Geometry: final body of the model. Coordinates: model frame, mm. Face numbers are marked on the shaded views. A direction names the side the tool comes from. Round coordinates to 2 decimals unless told otherwise and drop trailing zeros. Loops run counter-clockwise (first coordinate to the right, second up) from the corner with the lowest first, then second, coordinate; pieces in that order, holes last. Notation, with made-up numbers: M 27,-6 L 59,-6 A23 cw 59,29 Z; hole C 8,4.25 d9. An arc over 180 degrees is marked long. Write each question's results on one line, items separated by ' | '.
```python
from build123d import *

# Parameters (mm, degrees)
BOSS_EXTRUDE1_DEPTH = 40
SKETCH2_R           = 1.516102493
CUT_EXTRUDE1_DEPTH  = 10
SKETCH3_R           = 1.505855903
BOSS_EXTRUDE2_DEPTH = 5


with BuildPart() as part:
    # Sketch1 → Boss-Extrude1 (new body)
    with BuildSketch(Plane(origin=(0, 0, 0), x_dir=(1, 0, 0), z_dir=(0, 1, 0))):
        Polygon((0, -2.886751346), (2.5, -1.443375673), (2.5, 1.443375673), (0, 2.886751346), (-2.5, 1.443375673), (-2.5, -1.443375673), align=None)
    extrude(amount=BOSS_EXTRUDE1_DEPTH)

    # Sketch2 → Cut-Extrude1 (cut)
    with BuildSketch(Plane(origin=(0, 40, 0), x_dir=(1, 0, 0), z_dir=(0, 1, 0))):
        Circle(SKETCH2_R)
    extrude(amount=-CUT_EXTRUDE1_DEPTH, mode=Mode.SUBTRACT)

    # Sketch3 → Boss-Extrude2 (add)
    with BuildSketch(Plane.XZ):
        Circle(SKETCH3_R)
    extrude(amount=BOSS_EXTRUDE2_DEPTH)


solid = part.part
```
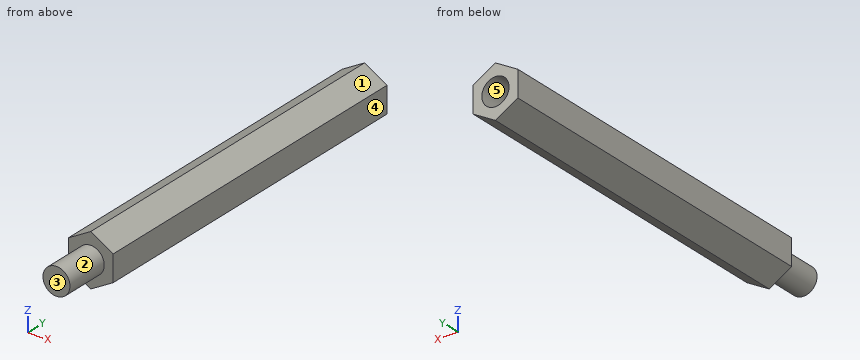
1. Draft query along X for the marked faces 3, 4 and 5. Return one class per face: pulls with the +X half, pulls with the -X half, needs draft (parallel to the pull), parting line crosses it, or undercut.
Answer key:
face 3: needs draft | face 4: pulls with the +X half | face 5: undercut
2. Section B-B (y = 31.5). Output: boundary loops of the cut face in (x, z).
Answer key:
outline: M -2.5,-1.44 L 0,-2.89 L 2.5,-1.44 L 2.5,1.44 L 0,2.89 L -2.5,1.44 Z; hole C 0,0 d3.03
3. Section A-A (z = 0). Output: boundary loops of the cut face in (x, y).
Answer key:
outline: M -2.5,0 L -1.51,0 L -1.51,-5 L 1.51,-5 L 1.51,0 L 2.5,0 L 2.5,40 L 1.52,40 L 1.52,30 L -1.52,30 L -1.52,40 L -2.5,40 Z
4. Section C-C (y = 21). Output: boundary loops of the cut face in (x, z).
Answer key:
outline: M -2.5,-1.44 L 0,-2.89 L 2.5,-1.44 L 2.5,1.44 L 0,2.89 L -2.5,1.44 Z
5. Pin query (flat end, axial travel): P1, Ø0.9, axis at x = -0.5, z = -0.5, coming from the +Y side; P2, Ø1, axis at x = -1, z = -2, coming from the -Y side. Return the tip coordinate at first contact, or that it passes through.
Answer key:
P1: stops at y = 30 | P2: stops at y = 0
6. Section D-D (x = -0.85). Output: boundary loops of the cut face in (y, z).
Answer key:
outline: M -5,-1.24 L 0,-1.24 L 0,-2.4 L 40,-2.4 L 40,-1.26 L 30,-1.26 L 30,1.26 L 40,1.26 L 40,2.4 L 0,2.4 L 0,1.24 L -5,1.24 Z
7. Ray query, probe 1 along X at (y, z) = (32.75, 0); probe 2 along Z at (x, y) = (0, 36.25); probe 3 along Y at (x, z) = (-0.3, -1.05). Return the intervals inside material, ascending.
Answer key:
probe 1: x = -2.5 to -1.52, 1.52 to 2.5 | probe 2: z = -2.89 to -1.52, 1.52 to 2.89 | probe 3: y = -5 to 30
8. Access query for the marked faces 1 and 2. Directions: +Z, -Z, +X, -X, +Y, -Y. A direction counts if a zero-diameter tool reaches every point of the face in a straight line with its end or side. Return the directions, or none.
Answer key:
face 1: +Z, +X, +Y, -Y | face 2: -Y
